from build123d import *

# Parameters (mm, degrees)
BOSS_EXTRUDE1_DEPTH = 18
SKETCH2_R           = 1.75
CUT_EXTRUDE1_DEPTH  = 31
CUT_EXTRUDE2_DEPTH  = 1
CUT_EXTRUDE3_DEPTH  = 5


with BuildPart() as part:
    # Sketch1 → Boss-Extrude1 (new body)
    with BuildSketch(Plane(origin=(0, 0, 0), x_dir=(1, 0, 0), z_dir=(0, 1, 0))):
        with BuildLine():
            ThreePointArc((-31.998275301, 18.509333542), (-46.998275301, -7.471428571), (-31.998275301, -33.452190685))
            Line((-31.998275301, -33.452190685), (-31.998275301, -47.471428571))
            Line((-31.998275301, -47.471428571), (-16.998275301, -47.471428571))
            Line((-16.998275301, -47.471428571), (-16.998275301, -30.471428571))
            ThreePointArc((-16.998275301, -30.471428571), (-39.998275301, -7.471428571), (-16.998275301, 15.528571429))
            Line((-16.998275301, 15.528571429), (-16.998275301, 32.528571429))
            Line((-16.998275301, 32.528571429), (-31.998275301, 32.528571429))
            Line((-31.998275301, 32.528571429), (-31.998275301, 18.509333542))
        make_face()
    extrude(amount=BOSS_EXTRUDE1_DEPTH)

    # Sketch2 → Cut-Extrude1 (cut, through all)
    with BuildSketch(Plane(origin=(-16.998275301, 0, 0), x_dir=(0, 0, -1), z_dir=(1, 0, 0))):
        with Locations((-42.471428571, 5.25)):
            Circle(SKETCH2_R)
        with Locations((27.528571429, 5.25)):
            Circle(SKETCH2_R)
    extrude(amount=-CUT_EXTRUDE1_DEPTH, mode=Mode.SUBTRACT)

    # Sketch3 → Cut-Extrude2 (cut)
    with BuildSketch(Plane(origin=(-16.998275301, 0, 0), x_dir=(0, 0, -1), z_dir=(1, 0, 0))):
        Polygon((-41.052726264, 15.110089197), (-38.474734811, 15.110089197), (-38.474734811, 14.160302873), (-40.102939939, 14.160302873), (-40.102939939, 13.142674667), (-38.474734811, 13.142674667), (-38.474734811, 12.192888343), (-40.102939939, 12.192888343), (-40.102939939, 9.818422531), (-41.052726264, 9.818422531), align=None)
        with BuildLine():
            Line((-36.914371563, 13.346200308), (-37.864157888, 13.346200308))
            add(Edge.make_bspline(
                [(-37.864157888, 13.346200308), (-37.860055906, 13.418046619), (-37.852040881, 13.558429997), (-37.820159135, 13.762341347), (-37.77743869, 13.955015151), (-37.720422585, 14.135777413), (-37.648778118, 14.304562451), (-37.564348886, 14.461945662), (-37.464977915, 14.60709842), (-37.352780144, 14.739320716), (-37.229660384, 14.857938558), (-37.098174722, 14.963112588), (-36.956311907, 15.049899551), (-36.806663889, 15.121317187), (-36.64925615, 15.178376559), (-36.482599366, 15.216525367), (-36.30813654, 15.242360114), (-36.188702609, 15.244620758), (-36.127829763, 15.245772958)],
                knots=[0, 0, 0, 0, 0.000215773, 0.000421607, 0.000618333, 0.000807411, 0.000989332, 0.001167669, 0.001342317, 0.001516048, 0.001686973, 0.001854511, 0.002020137, 0.00218466, 0.002351301, 0.002521253, 0.002696799, 0.002879275, 0.002879275, 0.002879275, 0.002879275], degree=3))
            add(Edge.make_bspline(
                [(-36.127829763, 15.245772958), (-36.053109208, 15.24344148), (-35.907237174, 15.238889888), (-35.695273537, 15.200063297), (-35.497322677, 15.135119825), (-35.313528483, 15.044376667), (-35.145455629, 14.929096996), (-34.993131985, 14.791644856), (-34.861164061, 14.629136428), (-34.748715142, 14.448333423), (-34.65528353, 14.256888487), (-34.589810548, 14.058926484), (-34.546775862, 13.859700523), (-34.542185946, 13.725551844), (-34.539905751, 13.658908976)],
                knots=[0, 0, 0, 0, 0.000224028, 0.000437354, 0.000643845, 0.000847219, 0.001050092, 0.001253455, 0.001460573, 0.001675861, 0.00189111, 0.002097935, 0.002300212, 0.002499903, 0.002499903, 0.002499903, 0.002499903], degree=3))
            add(Edge.make_bspline(
                [(-34.539905751, 13.658908976), (-34.540793539, 13.618598659), (-34.542580436, 13.537463948), (-34.555004968, 13.414687217), (-34.573644221, 13.289624762), (-34.601747672, 13.162383812), (-34.63679498, 13.032928701), (-34.679312431, 12.900872012), (-34.730286257, 12.76696246), (-34.788865811, 12.629692915), (-34.858751366, 12.488617716), (-34.940123382, 12.341622092), (-35.035141655, 12.188836439), (-35.142658484, 12.02939808), (-35.263196054, 11.863558473), (-35.397342788, 11.69181718), (-35.543553632, 11.513569038), (-35.64732358, 11.394420158), (-35.700637923, 11.333204515)],
                knots=[0, 0, 0, 0, 0.000120918, 0.000243377, 0.000369908, 0.000500063, 0.000634034, 0.000772147, 0.000916066, 0.001063745, 0.001219713, 0.001388155, 0.0015676, 0.00175929, 0.00196496, 0.002182512, 0.002412975, 0.002656496, 0.002656496, 0.002656496, 0.002656496], degree=3))
            Line((-35.700637923, 11.333204515), (-36.25291323, 10.700366975))
            Line((-36.25291323, 10.700366975), (-34.472063871, 10.700366975))
            Line((-34.472063871, 10.700366975), (-34.472063871, 9.818422531))
            Line((-34.472063871, 9.818422531), (-37.999841648, 9.818422531))
            Line((-37.999841648, 9.818422531), (-37.999841648, 10.299675869))
            Line((-37.999841648, 10.299675869), (-36.433118224, 11.967102085))
            add(Edge.make_bspline(
                [(-36.433118224, 11.967102085), (-36.387757555, 12.015741425), (-36.299907391, 12.109941403), (-36.17490566, 12.248284093), (-36.061790136, 12.379568004), (-35.962906361, 12.505191043), (-35.873065041, 12.621078512), (-35.796272194, 12.730723404), (-35.731825226, 12.833134488), (-35.661858901, 12.956624369), (-35.595413893, 13.103908028), (-35.534446576, 13.273584842), (-35.497282777, 13.435756798), (-35.492152997, 13.541431531), (-35.489692076, 13.592127125)],
                knots=[0, 0, 0, 0, 0.000199522, 0.000386415, 0.00055934, 0.00071926, 0.000865974, 0.000999188, 0.001120653, 0.001228864, 0.001424763, 0.001604456, 0.001769334, 0.001921366, 0.001921366, 0.001921366, 0.001921366], degree=3))
            add(Edge.make_bspline(
                [(-35.489692076, 13.592127125), (-35.491532047, 13.641171201), (-35.495097287, 13.736201961), (-35.534276384, 13.871382712), (-35.594974, 13.993775082), (-35.680505512, 14.09972185), (-35.784110962, 14.186785334), (-35.903836792, 14.251540708), (-36.038706883, 14.288904261), (-36.133253387, 14.293580844), (-36.181891261, 14.295986633)],
                knots=[0, 0, 0, 0, 0.000146748, 0.000284348, 0.000418508, 0.000554258, 0.000689709, 0.000822026, 0.000959626, 0.001105406, 0.001105406, 0.001105406, 0.001105406], degree=3))
            add(Edge.make_bspline(
                [(-36.181891261, 14.295986633), (-36.207018207, 14.295097906), (-36.256484634, 14.293348303), (-36.329196415, 14.281701669), (-36.3983869, 14.261175694), (-36.464826215, 14.233673776), (-36.527805303, 14.197219786), (-36.587165312, 14.152284435), (-36.643531673, 14.100009634), (-36.696645869, 14.040558837), (-36.74498672, 13.974211731), (-36.787922888, 13.90157426), (-36.823423951, 13.822691512), (-36.854680377, 13.738604861), (-36.878786828, 13.648411147), (-36.896339316, 13.552650169), (-36.909683299, 13.451477719), (-36.912780379, 13.381931173), (-36.914371563, 13.346200308)],
                knots=[0, 0, 0, 0, 7.5381e-05, 0.0001484, 0.000220186, 0.000291452, 0.000363636, 0.000437838, 0.000514351, 0.000593931, 0.00067662, 0.000760248, 0.000846574, 0.00093578, 0.001029123, 0.001126213, 0.001227716, 0.001334967, 0.001334967, 0.001334967, 0.001334967], degree=3))
        make_face()
    extrude(amount=-CUT_EXTRUDE2_DEPTH, mode=Mode.SUBTRACT)

    # Sketch4 → Cut-Extrude3 (cut)
    with BuildSketch(Plane.ZY.offset(31.998275301)):
        Polygon((-25.735714731, 2.629122629), (-24.362396696, 5.49222076), (-26.155253394, 8.113098131), (-29.321428126, 7.870877371), (-30.694746161, 5.00777924), (-28.901889463, 2.386901869), align=None)
        Polygon((45.170887067, 3.577798708), (45.269326619, 6.751698988), (42.569868123, 8.42390028), (39.771970075, 6.922201292), (39.673530524, 3.748301012), (42.37298902, 2.07609972), align=None)
    extrude(amount=-CUT_EXTRUDE3_DEPTH, mode=Mode.SUBTRACT)


solid = part.part
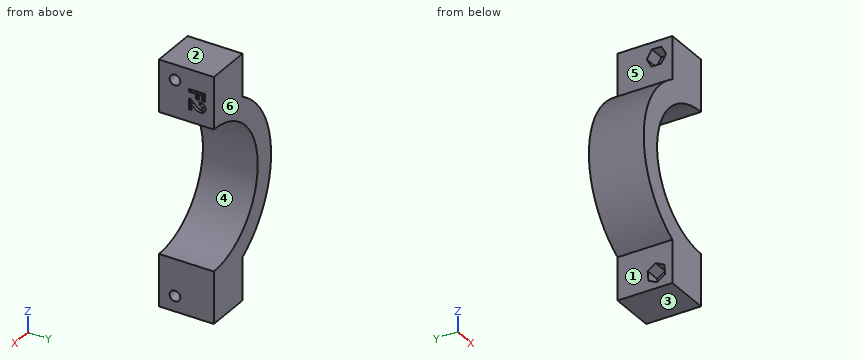
Could you check a few things on this model? Use its own coordinates, in mm. Face numbers are marked on the shaded views. A direction names the side the tool comes from. Round coordinates to 2 decimals unless told otherwise and drop trailing zeros. Loops run counter-clockwise (first coordinate to the right, second up) from the corner with the lowest first, then second, coordinate; pieces in that order, holes last. Notation, with made-up numbers: (31.5, -25) -> (76.5, -25) arc R21 cw to (76.5, -11) -> close; hole circle Ø7 at (73, 58). An arc over 180 degrees is marked (long way). Use CSV: the item, a comma, the result in double quotes.
(1) Suppose I cut it at A-A on x = -20. Write out the boundary of the cut face in (y, z), plus the area to 3 significant figures.
Return value:
outline,"(0, -32.53) -> (18, -32.53) -> (18, -15.33) -> (0, -15.33) -> close; (0, 30.27) -> (18, 30.27) -> (18, 47.47) -> (0, 47.47) -> close; hole circle Ø3.5 at (5.25, -27.53); hole circle Ø3.5 at (5.25, 42.47)"
area,"600 mm²"
(2) If I drill on probe 1 along Y at (x, z) = (-19.5, -28); probe 2 along Y at (x, z) = (-23.5, -27.5); probe 3 along X at (y, z) = (16.25, -26.5), over which ranges is the centre line in solid material (lowest first)? Write a range as [from, to].
Return value:
probe 1,"y = [0, 3.56], [6.94, 18]"
probe 2,"y = [0, 3.5], [7, 18]"
probe 3,"x = [-32, -17]"
(3) Will these pins go through, and if not, where does the flat tip stop? pin 1 Ø7 at (y, z) = (4.5, -22.5) entering from -X; pin 2 Ø1 at (y, z) = (11, 28.5) entering from -X; pin 3 Ø3 at (y, z) = (14, -11) entering from -X.
Return value:
pin 1,"stops at x = -32"
pin 2,"stops at x = -38.87"
pin 3,"stops at x = -41.74"
(4) Suppose I cut it at B-B on x = -34.5. Write out the boundary of the cut face in (y, z), plus the area to 3 significant figures.
Return value:
outline,"(0, -16.89) -> (18, -16.89) -> (18, -7.45) -> (0, -7.45) -> close; (0, 22.39) -> (18, 22.39) -> (18, 31.84) -> (0, 31.84) -> close"
area,"340 mm²"
(5) Suppose I cut it at C-C on z = 5.5. Write out the boundary of the cut face in (x, y), plus the area to 3 significant figures.
Return value:
outline,"(-46.93, 0) -> (-39.91, 0) -> (-39.91, 18) -> (-46.93, 18) -> close"
area,"126 mm²"
(6) If we mould it in two halves opening along Z, with no side actions, what happens to the marked faces 1, 2, 3 and 4? For each: +Z half, -Z half, draft (parallel to the pull), parting line (faces both ways), or undercut.
Return value:
face 1,"draft"
face 2,"+Z half"
face 3,"-Z half"
face 4,"undercut"
(7) Suppose I cut it at D-D on z = -4.5. Write out the boundary of the cut face in (x, y).
Return value:
outline,"(-44.51, 0) -> (-36.64, 0) -> (-36.64, 18) -> (-44.51, 18) -> close"
(8) For the marked faces 5 and 6, which set-ups out of +Z, -Z, +X, -X, +Y, -Y let a thin tool reach every point of the face, with its end or its side?
Return value:
face 5,"+Z, -X, +Y, -Y"
face 6,"+Z, -Z, +X, -X, +Y"
